from build123d import *

# Parameters (mm, degrees)
F0_W      = 26
F0_H      = 26
F0_W_2    = 16
F0_H_2    = 16
F1_DEPTH  = 2
F2_DEPTH  = 100
F3_W      = 26
F3_H      = 26
F3_W_2    = 18
F3_H_2    = 18
F4_DEPTH  = 4
F5_W      = 5
F5_H      = 4
F6_DEPTH  = 4
F7_D      = 2.7
F7_DEPTH  = 4
F7_TIP    = 0.8111618357
F9_W      = 3
F9_H      = 16
F10_DEPTH = 26
F11_W     = 4
F11_H     = 12
F12_DEPTH = 20
F13_W     = 16
F13_H     = 15
F14_DEPTH = 40


with BuildPart() as f1:
    # F0 (on Top) → F1 (new body)
    with BuildSketch(Plane.XY):
        Rectangle(F0_W, F0_H)
        Rectangle(F0_W_2, F0_H_2, mode=Mode.SUBTRACT)
        Rectangle(F0_W_2, F0_H_2)
    extrude(amount=F1_DEPTH)

    # F0 (on Top) → F2 (join)
    with BuildSketch(Plane.XY):
        Rectangle(F0_W, F0_H)
        Rectangle(F0_W_2, F0_H_2, mode=Mode.SUBTRACT)
    extrude(amount=F2_DEPTH)

    # F3 (on face) → F4 (join)
    with BuildSketch(Plane.XY.offset(100)):
        Rectangle(F3_W, F3_H)
        Rectangle(F3_W_2, F3_H_2, mode=Mode.SUBTRACT)
    extrude(amount=F4_DEPTH)

    # F5 (on face) → F6 (cut, through all)
    with BuildSketch(Plane.XY.offset(104)):
        with Locations((0, -11)):
            Rectangle(F5_W, F5_H)
        with Locations((0, 11)):
            Rectangle(F5_W, F5_H)
    extrude(amount=-F6_DEPTH, mode=Mode.SUBTRACT)

    # F7
    with Locations(Plane.XY.offset(104)):
        with Locations((-10.5, 10.5), (10.5, 10.5), (-10.5, -10.5), (10.5, -10.5)):
            Hole(F7_D / 2, depth=F7_DEPTH)
            with Locations((0, 0, -(F7_DEPTH + F7_TIP / 2))):  # 118° drill point
                Cone(0, F7_D / 2, F7_TIP, mode=Mode.SUBTRACT)

    # F9 (on face) → F10 (join)
    with BuildSketch(Plane.XZ.offset(13)):
        with Locations((-14.5, 63)):
            Rectangle(F9_W, F9_H)
    extrude(amount=-F10_DEPTH)

    # F11 (on face) → F12 (cut)
    with BuildSketch(Plane.XZ.offset(13)):
        with Locations((-9, 63)):
            Rectangle(F11_W, F11_H)
    extrude(amount=-F12_DEPTH, mode=Mode.SUBTRACT)

    # F13 (on face) → F14 (join)
    with BuildSketch(Plane.XZ.offset(13)):
        with Locations((0, 9.5)):
            Rectangle(F13_W, F13_H)
    extrude(amount=-F14_DEPTH)


solid = f1.part
Can you work these out from the model? Positions are in its coordinate system, mm. A direction names the side the tool comes from. Give positions to 0.01 mm unless a question says otherwise; leave off trailing zeros. Order: outer loops, then holes, each group sorted by start corner. A loop starts at its lowest first (then second) coordinate and runs counter-clockwise, first axis right, second up. Notation, with made-up numbers: M 20.5,33.25 L 71.5,33.25 A18 cw 71.5,54.25 Z; hole C 38.25,74 d8. An arc over 180 degrees is marked long. Use one line per item in the form item = value. Start each with the question number.
Item 1: Will these pins go through, and if not, where does the flat tip stop? pin 1 Ø12 at (y, z) = (22.5, 84.5) entering from -X; pin 2 Ø4 at (x, z) = (1.5, 44) entering from +Y; pin 3 Ø5 at (y, z) = (0, 52) entering from -X; pin 4 Ø3 at (x, y) = (4, 18) entering from +Z.
Item 2: For faces 4 (the flat face through (-13, 0, 87)), 5 (the flat face through (8, 0, 58)), 6 (the flat face through (-13, 0, 27)), 7 (the flat face through (-7, -11, 63)), 8 (the flat face through (0, 20, 2)), which set-ups out of +Z, -Z, +X, -X, +Y, -Y let a thin tool reach every point of the face, with its end or its side?
Item 3: We'd pull the mould along Z, two halves only. Please class faces 1 (the flat face through (-8, 20, 9)), 2 (the conical face through (10.72, -10.59, 99.33)), 3 (the flat face through (-10, 7, 63)): +Z half, -Z half, draft (parallel to the pull), parting line (faces both ways), or undercut.
Item 4: If we section it at C-C (y = 17): Write out the boundary of the cut face in (x, z).
Item 5: If we section it at D-D (x = 7): Write out the boundary of the cut face in (y, z), then the cut area to 3 significant figures.
Item 6: If we section it at A-A (z = 37): Write out the boundary of the cut face in (x, y), then the cut area to 3 significant figures.
Item 7: If we section it at B-B (x = 0): Write out the boundary of the cut face in (y, z).
Item 8: If I drill on line 1 along Y through (x, z) = (-10.5, 101.85); line 2 along X through (y, z) = (10.5, 101.5); line 3 along Y through (x, z) = (-6.5, 52), over which ranges is the centre line in solid material (lowest first)?
Outcome:
q1.pin_1 = through
q1.pin_2 = 13
q1.pin_3 = -13
q1.pin_4 = 17
q2.face_4 = +Z, -X, +Y, -Y
q2.face_5 = +Z
q2.face_6 = -Z, -X, +Y, -Y
q2.face_7 = -Y
q2.face_8 = -Z, +X, -X, +Y
q3.face_1 = draft
q3.face_2 = +Z half
q3.face_3 = undercut
q4.outline = M -8,2 L 8,2 L 8,17 L -8,17 Z
q5.outline = M -13,0 L 13,0 L 13,2 L 27,2 L 27,17 L 13,17 L 13,104 L 9,104 L 9,100 L 8,100 L 8,17 L -8,17 L -8,100 L -9,100 L -9,104 L -13,104 Z
q5.area = 1,510 mm2
q6.outline = M -13,-13 L 13,-13 L 13,13 L -13,13 Z; hole M -8,-8 L 8,-8 L 8,8 L -8,8 Z
q6.area = 420 mm2
q7.outline = M -13,0 L 13,0 L 13,2 L 27,2 L 27,17 L 13,17 L 13,100 L 8,100 L 8,17 L -8,17 L -8,100 L -13,100 Z
q8.line_1 = -13 to -11.85, -9.15 to 9.15, 11.85 to 13
q8.line_2 = -13 to -11.85, -9.15 to -2.5, 2.5 to 9.15, 11.85 to 13
q8.line_3 = -13 to -8, 8 to 13
